```python
from build123d import *

# Parameters (mm, degrees)
BOSS_EXTRUDE1_DEPTH = 120
SKETCH2_R           = 87.5
CUT_EXTRUDE1_DEPTH  = 120
SKETCH3_R           = 25
CUT_EXTRUDE2_DEPTH  = 120
SHELL2_START        = 12
SHELL2_OUTLINE_R    = 25
SHELL2_DEPTH        = 96
CUT_EXTRUDE4_DEPTH  = 120
CUT_EXTRUDE5_DEPTH  = 120
BOSS_EXTRUDE2_DEPTH = 10
BOSS_EXTRUDE3_DEPTH = 10
FILLET1_R           = 8


# Read off the part's stored shape, not the designer's step: Shell2
with BuildPart() as part:
    # Sketch1 → Boss-Extrude1 (new body)
    with BuildSketch(Plane.XY):
        with BuildLine():
            Line((-105.840625, 29.962678445), (0, 792.401413426))
            ThreePointArc((0, 792.401413426), (69.989991069, 814.210311801), (67.715560492, 740.936483843))
            Line((67.715560492, 740.936483843), (67.715560492, 126.004465834))
            Line((67.715560492, 126.004465834), (87.732689968, 66.35491776))
            ThreePointArc((87.732689968, 66.35491776), (20.324199821, -108.106090955), (-105.840625, 29.962678445))
        make_face()
    extrude(amount=BOSS_EXTRUDE1_DEPTH)

    # Sketch2 → Cut-Extrude1 (cut)
    with BuildSketch(Plane.XY.offset(120)):
        Circle(SKETCH2_R)
    extrude(amount=-CUT_EXTRUDE1_DEPTH, mode=Mode.SUBTRACT)

    # Sketch3 → Cut-Extrude2 (cut)
    with BuildSketch(Plane.XY.offset(120)):
        with Locations((42.760873913, 778.383294358)):
            Circle(SKETCH3_R)
    extrude(amount=-CUT_EXTRUDE2_DEPTH, mode=Mode.SUBTRACT)

    # Shell2 outline → Shell2 (cut)
    with BuildSketch(Plane.XY.offset(SHELL2_START)):
        with BuildLine():
            Line((75.655144686, 64.626225966), (55.715560492, 124.0446949))
            Line((55.715560492, 124.0446949), (55.715560492, 748.032411411))
            ThreePointArc((55.715560492, 748.032411411), (65.426599219, 802.367974809), (11.726520361, 789.602425324))
            Line((11.726520361, 789.602425324), (-92.959881421, 35.478309517))
            ThreePointArc((-92.959881421, 35.478309517), (-16.948856501, 98.045837562), (75.655144686, 64.626225966))
        make_face()
        with Locations((42.760873913, 778.383294358)):
            Circle(SHELL2_OUTLINE_R, mode=Mode.SUBTRACT)
    extrude(amount=SHELL2_DEPTH, mode=Mode.SUBTRACT)

    # Sketch4 → Cut-Extrude4 (cut)
    with BuildSketch(Plane.XY.offset(120)):
        with BuildLine():
            Line((-54.201038132, 110.893822017), (46.63374807, 242.267143469))
            ThreePointArc((46.63374807, 242.267143469), (52.207619727, 243.957335897), (55.600099295, 239.222794941))
            Line((55.600099295, 239.222794941), (55.600099295, 106.065561115))
            ThreePointArc((55.600099295, 106.065561115), (53.272224451, 101.839481708), (48.456200434, 101.548515878))
            add(Edge.make_bspline(
                [(-48.203411652, 103.280674868), (-32.29772345, 110.352299936), (0.49057596, 117.216976021), (32.14071495, 109.29223969), (48.456200434, 101.548515878)],
                knots=[0.164763499, 0.164763499, 0.164763499, 0.164763499, 0.551333425, 0.942878972, 0.942878972, 0.942878972, 0.942878972], degree=3))
            ThreePointArc((-48.203411652, 103.280674868), (-54.162298411, 104.755306741), (-54.201038132, 110.893822017))
        make_face()
        with BuildLine():
            Line((-53.553065242, 253.949018208), (33.287473267, 253.949018208))
            ThreePointArc((33.287473267, 253.949018208), (37.771987881, 251.160155626), (37.253824493, 245.90466968))
            Line((37.253824493, 245.90466968), (-70.005272034, 106.161389635))
            ThreePointArc((-70.005272034, 106.161389635), (-75.918077174, 104.600163589), (-78.919089143, 109.928636031))
            Line((-78.919089143, 109.928636031), (-58.500531126, 249.671916076))
            ThreePointArc((-58.500531126, 249.671916076), (-56.823043121, 252.731510068), (-53.553065242, 253.949018208))
        make_face()
        with BuildLine():
            Line((-52.732234928, 278.037445865), (31.376208078, 278.037445865))
            ThreePointArc((31.376208078, 278.037445865), (35.555871549, 280.293286019), (35.964073946, 285.02528056))
            Line((35.964073946, 285.02528056), (-27.226737743, 430.86787452))
            ThreePointArc((-27.226737743, 430.86787452), (-32.478658579, 433.835746738), (-36.76395609, 429.589906043))
            Line((-36.76395609, 429.589906043), (-57.681587406, 283.747312082))
            ThreePointArc((-57.681587406, 283.747312082), (-56.510417764, 279.762490223), (-52.732234928, 278.037445865))
        make_face()
        with BuildLine():
            Line((-14.009585394, 447.087418489), (47.46310653, 447.087418489))
            ThreePointArc((47.46310653, 447.087418489), (50.998640436, 445.622952394), (52.46310653, 442.087418489))
            Line((52.46310653, 442.087418489), (52.46310653, 300.210196021))
            ThreePointArc((52.46310653, 300.210196021), (48.478160878, 295.314313601), (42.875240662, 298.222361327))
            Line((42.875240662, 298.222361327), (-18.597451263, 440.099583794))
            ThreePointArc((-18.597451263, 440.099583794), (-18.189248866, 444.831578335), (-14.009585394, 447.087418489))
        make_face()
    extrude(amount=-CUT_EXTRUDE4_DEPTH, mode=Mode.SUBTRACT)

    # Sketch6 → Cut-Extrude5 (cut)
    with BuildSketch(Plane(origin=(67.715560492, 0, 0), x_dir=(0, 0, -1), z_dir=(1, 0, 0))):
        Polygon((-120, 480.355293397), (-115, 492.394948365), (-115, 740.936483843), (-120, 740.936483843), align=None)
        Polygon((0, 740.936483843), (-5, 740.936483843), (-5, 492.394948365), (0, 480.355293397), align=None)
    extrude(amount=-CUT_EXTRUDE5_DEPTH, mode=Mode.SUBTRACT)

    # Sketch9 → Boss-Extrude2 (add)
    with BuildSketch(Plane(origin=(0, 0, 5), x_dir=(-1, 0, 0), z_dir=(0, 0, -1))):
        Polygon((-52.957009084, 634.164562087), (5.972067956, 634.164562087), (23.731094104, 506.234767355), (-52.957009084, 506.234767355), align=None)
    extrude(amount=BOSS_EXTRUDE2_DEPTH)

    # Sketch7 → Boss-Extrude3 (add)
    with BuildSketch(Plane.XY.offset(115)):
        Polygon((-5.972067956, 634.164562087), (52.957009084, 634.164562087), (52.957009084, 506.234767355), (-23.731094104, 506.234767355), align=None)
    extrude(amount=BOSS_EXTRUDE3_DEPTH)

    # Fillet1
    fillet1_edges = [part.edges().sort_by_distance(p)[0] for p in [
        (52.957009084, 570.199664721, -5),
        (14.61295749, 506.234767355, -5),
        (-14.85158103, 570.199664721, -5),
        (23.492470564, 634.164562087, -5),
        (-14.85158103, 570.199664721, 125),
        (14.61295749, 506.234767355, 125),
        (52.957009084, 570.199664721, 125),
        (23.492470564, 634.164562087, 125),
    ]]
    fillet(fillet1_edges, radius=FILLET1_R)


solid = part.part
```
CAD build for the part. Positions are in the model's coordinates, mm. A direction names the side the tool comes from. Round coordinates to 2 decimals unless told otherwise and drop trailing zeros. Order: outer loops, then holes, each group sorted by start corner. A loop starts at its lowest first (then second) coordinate and runs counter-clockwise, first axis right, second up. Notation, with made-up numbers: (-12, 22) -> (-4, 22) arc R27 cw to (-4, 57) -> close; hole circle Ø11 at (37.5, -15). An arc over 180 degrees is marked (long way). One line per question, with ' | ' between items.
Q1. Which spindle directions (+Z, -Z, +X, -X, +Y, -Y) get a long thin tool onto all of the face, cutting with end or side? Do faces 5 (the flat face through (16, 483, 12)), 6 (the flat face through (-47.076, 357.69, 114.084)), 7 (the flat face through (1, 187, 120)). Say none if no direction does.
Completed:
face 5: none | face 6: +Z, -Z | face 7: +Z, +X, -X, -Y
Q2. Two-plate mould, pull along Z, no slides. Class faces 1 (the cylindrical face through (-12.47, 570.78, 122.59)), 2 (the flat face through (-14.976, 569.304, 115.986)), 3 (the flat face through (20, 792, 0)), 4 (the cylindrical face through (66.083, 801.73, 59.328)): released by +Z, released by -Z, zero draft, split by the parting line, or undercut.
Completed:
face 1: released by +Z | face 2: zero draft | face 3: released by -Z | face 4: undercut
Q3. Slice it at B-B (z = 49.5). Write the cut outline in (x, y), then the cut area to 3 significant figures.
Completed:
outline: (-105.84, 29.96) arc R110 ccw (long way) to (87.73, 66.35) -> (67.72, 126) -> (67.72, 740.94) arc R45 ccw (long way) to (0, 792.4) -> close; hole (-92.96, 35.48) arc R99.5 cw to (75.66, 64.63) -> (55.72, 124.04) -> (55.72, 748.03) arc R33 ccw (long way) to (11.73, 789.6) -> close; hole circle Ø175 at (0, 0) | area: 30,800 mm^2
Q4. Slice it at A-A (y = 0). Write the cut outline in (x, z).
Completed:
outline: (-110, 0) -> (-87.5, 0) -> (-87.5, 120) -> (-110, 120) -> close; (87.5, 0) -> (110, 0) -> (110, 120) -> (87.5, 120) -> close
Q5. Slice it at D-D (y = 648.5). Write the cut outline in (x, z), then the cut area to 3 significant figures.
Completed:
outline: (-19.98, 5) -> (67.72, 5) -> (67.72, 115) -> (-19.98, 115) -> close; hole (-7.86, 12) -> (55.72, 12) -> (55.72, 108) -> (-7.86, 108) -> close | area: 3,540 mm^2
Q6. Drop flat-ended pins along their axis: pin 1 (4 mm diameter, centred on y = 326, z = 19, fed in from -X); pin 2 (6 mm diameter, centred on x = -83, y = 93, fed in from +Z); pin 3 (5 mm diameter, centred on x = 72.5, z = 91.5, fed in from -Y). Give the stop position or say it passes through.
Completed:
pin 1: stops at x = -65.02 | pin 2: stops at z = 120 | pin 3: stops at y = -84.85
Q7. Slice it at C-C (y = 140). Write the cut outline in (x, z).
Completed:
outline: (-90.57, 0) -> (-74.53, 0) -> (-74.53, 12) -> (-78.45, 12) -> (-78.45, 108) -> (-74.53, 108) -> (-74.53, 120) -> (-90.57, 120) -> close; (-44.03, 0) -> (-31.86, 0) -> (-31.86, 12) -> (-44.03, 12) -> close; (-44.03, 108) -> (-31.86, 108) -> (-31.86, 120) -> (-44.03, 120) -> close; (55.6, 0) -> (67.72, 0) -> (67.72, 120) -> (55.6, 120) -> (55.6, 108) -> (55.72, 108) -> (55.72, 12) -> (55.6, 12) -> close
Q8. Probe probe 1 along Z at (x, y) = (31.5, 270); probe 2 along Z at (x, y) = (-75.5, -60); probe 3 along Z at (x, y) = (-1.5, 579). List the from-to ranges inside material, lowest first.
Completed:
probe 1: z = 0 to 12, 108 to 120 | probe 2: z = 0 to 120 | probe 3: z = -5 to 12, 108 to 125
